Geometry: final body of the model. Coordinates: model frame, mm. A direction names the side the tool comes from. Give positions to 0.01 mm unless a question says otherwise; leave off trailing zeros. Order: outer loops, then holes, each group sorted by start corner. A loop starts at its lowest first (then second) coordinate and runs counter-clockwise, first axis right, second up. Notation, with made-up numbers: M -37,74.25 L -12,74.25 A16 ccw -12,103.25 Z; hole C 64,5 d7. An arc over 180 degrees is marked long. Use CSV: the item, a comma, the result in double quotes.
```python
from build123d import *
from build123d.topology import SkipClean

# Parameters (mm, degrees)
SKETCH4_R           = 25.4
SKETCH4_R_2         = 20.32
BOSS_EXTRUDE1_DEPTH = 11.684
CHAMFER1_SIZE       = 1.27
THREAD3_PITCH       = 6.35
CUT_EXTRUDE2_DEPTH  = 64.791431358
SKETCH19_R          = 16.51
CUT_EXTRUDE3_DEPTH  = 4.318
SKETCH21_R          = 36.83
SKETCH21_R_2        = 25.4
BOSS_EXTRUDE2_DEPTH = 0.762


with BuildPart() as part:
    # Sketch1 → Revolve1 (revolve)
    with BuildSketch(Plane(origin=(0, 0, 0), x_dir=(1, 0, 0), z_dir=(0, 1, 0))):
        with BuildLine():
            Line((0, 0), (0, 36.83))
            ThreePointArc((0, 36.83), (-26.042742751, 26.042742751), (-36.83, 0))
            Line((-36.83, 0), (0, 0))
        make_face()
    revolve(axis=Axis((0, 0, 0), (0, 0, -1)))

    # Sketch4 → Boss-Extrude1 (add)
    with BuildSketch(Plane.XY):
        with Locations(Location((0, 0, 0), (0, 0, 180))):
            Circle(SKETCH4_R)
        Circle(SKETCH4_R_2, mode=Mode.SUBTRACT)
    extrude(amount=BOSS_EXTRUDE1_DEPTH)

    # Chamfer1
    chamfer1_edges = [part.edges().sort_by_distance(p)[0] for p in [
        (25.4, 0, 11.684),
    ]]
    chamfer(chamfer1_edges, length=CHAMFER1_SIZE)

    # Thread3: the profile of Thread Profile4 profile screwed along a right-hand helix of 1.84 turns, 14 arcs to a turn; built about Z, then put on its axis
    with SkipClean():  # the faces are left unmerged after this step: merging them gives an invalid solid
        thread3_z = Axis((0, 0, 0), (0, 0, 1))
        thread3_corners = [(25.4003, 0, -0.000173205), (25.4003, 0, 5.556423188), (21.962961694, 0, 3.571874991), (21.962961694, 0, 1.984374991)]
        with BuildLine(mode=Mode.PRIVATE) as thread3_profile:
            Line(thread3_corners[0], thread3_corners[1])
            Line(thread3_corners[1], thread3_corners[2])
            Line(thread3_corners[2], thread3_corners[3])
            Line(thread3_corners[3], thread3_corners[0])
        thread3_cap = Face(thread3_profile.wire())
        thread3_turn_angles = [0, 12.857142857, 25.714285714, 38.571428571, 51.428571429, 64.285714286, 77.142857143, 90, 102.857142857, 115.714285714, 128.571428571, 141.428571429, 154.285714286, 167.142857143, 180, 192.857142857, 205.714285714, 218.571428571, 231.428571429, 244.285714286, 257.142857143, 270, 282.857142857, 295.714285714, 308.571428571, 321.428571429, 334.285714286, 347.142857143, 360]
        thread3_turn_weights = [1, 0.9749279121818236, 1, 0.9749279121818236, 1, 0.9749279121818236, 1, 0.9749279121818236, 1, 0.9749279121818236, 1, 0.9749279121818236, 1, 0.9749279121818236, 1, 0.9749279121818236, 1, 0.9749279121818236, 1, 0.9749279121818236, 1, 0.9749279121818236, 1, 0.9749279121818237, 1, 0.9749279121818236, 1, 0.9749279121818236, 1]
        thread3_turn_rails = [Edge.make_bspline([Vector(p[0], p[1], 0).rotate(thread3_z, thread3_turn_angles[k]) / thread3_turn_weights[k] + Vector(0, 0, p[2] + THREAD3_PITCH * thread3_turn_angles[k] / 360) for k in range(29)], [0, 0, 0, 1, 1, 2, 2, 3, 3, 4, 4, 5, 5, 6, 6, 7, 7, 8, 8, 9, 9, 10, 10, 11, 11, 12, 12, 13, 13, 14, 14, 14], 2, thread3_turn_weights) for p in thread3_corners]
        thread3_turn_sides = [Face.make_surface_from_curves(thread3_turn_rails[p[0]], thread3_turn_rails[p[1]]) for p in [(0, 1), (1, 2), (2, 3), (3, 0)]]
        thread3_last_angles = [360, 372.857142857, 385.714285714, 398.571428571, 411.428571429, 424.285714286, 437.142857143, 450, 462.857142857, 475.714285714, 488.571428571, 501.428571429, 514.285714286, 527.142857143, 540, 552.857142857, 565.714285714, 578.571428571, 591.428571429, 604.285714286, 617.142857143, 630, 642.857142857, 652.628571429, 662.4]
        thread3_last_weights = [1, 0.9749279121818236, 1, 0.9749279121818236, 1, 0.9749279121818237, 1, 0.9749279121818235, 1, 0.9749279121818237, 1, 0.9749279121818237, 1, 0.9749279121818235, 1, 0.9749279121818235, 1, 0.9749279121818237, 1, 0.9749279121818237, 1, 0.9749279121818235, 1, 0.9854926535657266, 1]
        thread3_last_rails = [Edge.make_bspline([Vector(p[0], p[1], 0).rotate(thread3_z, thread3_last_angles[k]) / thread3_last_weights[k] + Vector(0, 0, p[2] + THREAD3_PITCH * thread3_last_angles[k] / 360) for k in range(25)], [0, 0, 0, 1, 1, 2, 2, 3, 3, 4, 4, 5, 5, 6, 6, 7, 7, 8, 8, 9, 9, 10, 10, 11, 11, 12, 12, 12], 2, thread3_last_weights) for p in thread3_corners]
        thread3_last_sides = [Face.make_surface_from_curves(thread3_last_rails[p[0]], thread3_last_rails[p[1]]) for p in [(0, 1), (1, 2), (2, 3), (3, 0)]]
        thread3 = Plane(origin=(0, 0, 0), x_dir=(1, 0, 0), z_dir=(0, 0, 1)) * Solid(Shell([*thread3_turn_sides, *thread3_last_sides, thread3_cap, thread3_cap.rotate(thread3_z, 662.4).moved(Location((0, 0, THREAD3_PITCH * 662.4 / 360)))]))
        add(thread3, mode=Mode.SUBTRACT)

    # Sketch18 → Cut-Extrude2 (cut, through all)
    with SkipClean():  # the faces are left unmerged after this step: merging them gives an invalid solid
        with BuildSketch(Plane(origin=(0, 0, 0), x_dir=(1, 0, 0), z_dir=(0, 1, 0))):
            Polygon((25.4, 0), (21.962961694, -1.984374991), (21.962961694, -3.571874991), (25.4, -5.556249983), align=None)
        extrude(amount=-CUT_EXTRUDE2_DEPTH, mode=Mode.SUBTRACT)

    # Sketch19 → Cut-Extrude3 (cut)
    with SkipClean():  # the faces are left unmerged after this step: merging them gives an invalid solid
        with BuildSketch(Plane.XY):
            Circle(SKETCH19_R)
        extrude(amount=-CUT_EXTRUDE3_DEPTH, mode=Mode.SUBTRACT)

    # Sketch21 → Boss-Extrude2 (add)
    with SkipClean():  # the faces are left unmerged after this step: merging them gives an invalid solid
        with BuildSketch(Plane.XY):
            with Locations(Location((0, 0, 0), (0, 0, 180))):
                Circle(SKETCH21_R)
            Circle(SKETCH21_R_2, mode=Mode.SUBTRACT)
        extrude(amount=BOSS_EXTRUDE2_DEPTH)


solid = part.part
```
1. Line query: line 1 (Y direction, x = 0, z = -1); line 2 (X direction, y = -4.5, z = -3.5); line 3 (Y direction, x = 0, z = 9). Output: solid intervals per line, ascending.
Answer:
line 1,"-36.82 to -16.51, 16.51 to 36.82"
line 2,"-36.39 to -15.88, 15.88 to 36.39"
line 3,"-23.12 to -20.32, 20.32 to 23.56"
2. Section D-D, the plane z = -11.5. Return the cut outline in (x, y), plus the area to 3 significant figures.
Answer:
outline,"C 0,0 d69.98"
area,"3,850 mm2"
3. Reachability of faces 5 (the face through (29.227, 22.41, 0.376)), 6 (the face through (-2.645, 20.147, 5.76)), 7 (the face through (23.28, -4.87, 4.33)) from +Z, -Z, +X, -X, +Y, -Y: full face, straight path, thin tool, end or side. Return the list, or none.
Answer:
face 5,"+Z, -Z"
face 6,"+Z"
face 7,"+X, +Y, -Y"
4. Section C-C, the plane z = -1. Return the cut outline in (x, y), plus the area to 3 significant figures.
Answer:
outline,"C 0,0 d73.63; hole C 0,0 d33.02"
area,"3,400 mm2"
5. Pin query (flat end, axial travel): pin 1 Ø4 at (x, z) = (-24, 2.5) entering from +Y; pin 2 Ø2 at (x, y) = (-19.5, 16.5) entering from +Z; pin 3 Ø12 at (y, z) = (-5.5, -10.5) entering from -X. Return the tip coordinate at first contact, or that it passes through.
Answer:
pin 1,"y = 28.76"
pin 2,"z = 9.31"
pin 3,"x = -36.36"
6. Section A-A, the plane z = -20.5. Return the cut outline in (x, y).
Answer:
outline,"C 0,0 d61.19"
7. Pull-direction query (X, two-part tool) for faces 1 (the face through (20, -4.4, 11.684)), 2 (the face through (23.32, -4.87, 1.2)), 3 (the face through (8.704, -22.723, 11.481)), 4 (the face through (0, 0, -4.318)); classes: +X half, -X half, draft (parallel to the pull), parting line (faces both ways), or undercut.
Answer:
face 1,"draft"
face 2,"undercut"
face 3,"parting line"
face 4,"undercut"
8. Section B-B, the plane y = 31. Return the cut outline in (x, z).
Answer:
outline,"M -19.89,0 A19.89 ccw 19.89,0 L 19.89,0.76 L -19.89,0.76 Z"
